Geometry check sheet. Reference: the model listing, model coordinates, mm. Face numbers are marked on the shaded views. Coordinates: 2 decimals unless noted, no trailing zeros. Order: outer loops, then holes, each group sorted by start corner. A loop starts at its lowest first (then second) coordinate and runs counter-clockwise, first axis right, second up. Notation, with made-up numbers: M 27.25,-27.75 L 72.25,-27.75 A11 cw 72.25,-10.75 Z; hole C 80.5,-19 d5. An arc over 180 degrees is marked long. One line per item, written item: value. Start each with the question number.
1) Thickness scan on L1, parallel to Z at x = -60.5, y = 8; L2, parallel to Z at x = -73, y = 5.5; L3, parallel to Y at x = -23.5, z = -3.5. Record the ranges inside material, lowest first. Write a range as from..to.
2) Sectioned sample at B-B, the plane z = -13.75. Enter the section's corners in (x, y), then the cut area to 3 significant figures.
3) Go/stop test with flat-tipped pins: P1, Ø12, axis at x = 75.5, y = -13.5, coming from the -Z side; P2, Ø2.5, axis at x = -84.5, y = 21, coming from the -Z side; P3, Ø3.5, axis at x = -101, y = -3.5, coming from the +Z side. Record where each tip stops, or that it passes through.
4) Draft check along X on the marked faces 1, 2 and 3. Enter one of: pulls with the +X half, pulls with the -X half, needs draft (parallel to the pull), parting line crosses it, or undercut.
5) Sectioned sample at A-A, the plane z = 0. Enter the section's corners in (x, y), then the cut area to 3 significant figures.
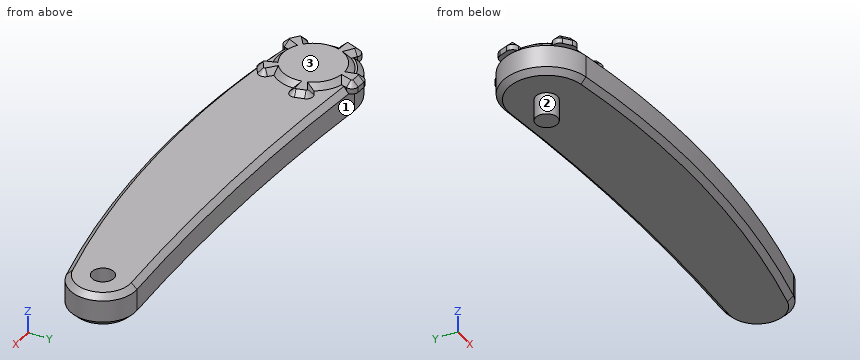
```python
from build123d import *

# Parameters (mm, degrees)
BOSS_EXTRUDE2_DEPTH = 7.5
CHAMFER1_SIZE       = 2.5
SKETCH4_R           = 16.5
BOSS_EXTRUDE3_DEPTH = 2.5
BOSS_EXTRUDE4_DEPTH = 5
CHAMFER2_SIZE       = 2.5
SKETCH6_R           = 5
CUT_EXTRUDE1_DEPTH  = 10
SKETCH7_R           = 5
BOSS_EXTRUDE5_DEPTH = 10


with BuildPart() as part:
    # Sketch1 → Boss-Extrude2 (new, symmetric)
    with BuildSketch(Plane.XY):
        with BuildLine():
            ThreePointArc((84.460518945, 14.977598104), (0.616073919, 13.910903957), (-83.022979725, 19.872238008))
            ThreePointArc((-83.022979725, 19.872238008), (-105.080474764, 2.818038301), (-88.656802688, -19.712869593))
            ThreePointArc((-88.656802688, -19.712869593), (0.254242747, -25.987416271), (88.657894096, -14.614713664))
            ThreePointArc((88.657894096, -14.614713664), (100.131353297, 2.106516275), (84.460518945, 14.977598104))
        make_face()
    extrude(amount=BOSS_EXTRUDE2_DEPTH, both=True)

    # Chamfer1
    chamfer1_edges = [part.edges().sort_by_distance(p)[0] for p in [
        (100.131353297, 2.106516275, 7.5),
        (0.616073919, 13.910903957, 7.5),
        (-105.080474764, 2.818038301, 7.5),
        (0.254242747, -25.987416271, 7.5),
        (-105.080474764, 2.818038301, -7.5),
        (0.616073919, 13.910903957, -7.5),
        (100.131353297, 2.106516275, -7.5),
        (0.254242747, -25.987416271, -7.5),
    ]]
    chamfer(chamfer1_edges, length=CHAMFER1_SIZE)

    # Sketch4 → Boss-Extrude3 (add, symmetric)
    with BuildSketch(Plane.XY.offset(7.5)):
        with Locations((-85.280003554, 0)):
            Circle(SKETCH4_R)
    extrude(amount=BOSS_EXTRUDE3_DEPTH, both=True)

    # Sketch5 → Boss-Extrude4 (add)
    with BuildSketch(Plane.XY.offset(10)):
        with BuildLine():
            Line((-68.665882393, 9.592167325), (-85.280003554, 0))
            Line((-85.280003554, 0), (-66.095668905, 0))
            ThreePointArc((-66.095668905, 0), (-63.715608884, 1.173715713), (-63.197891426, 3.776457135))
            Line((-63.197891426, 3.776457135), (-64.268104914, 7.770548248))
            ThreePointArc((-64.268104914, 7.770548248), (-66.017832096, 9.765729711), (-68.665882393, 9.592167325))
        make_face()
        with BuildLine():
            Line((-71.023264529, -12.836825476), (-85.280003554, 0))
            Line((-85.280003554, 0), (-79.351718121, -18.245386479))
            ThreePointArc((-79.351718121, -18.245386479), (-77.49996915, -20.146259969), (-74.864631467, -19.834347199))
            Line((-74.864631467, -19.834347199), (-71.396739243, -17.582271657))
            ThreePointArc((-71.396739243, -17.582271657), (-70.039904347, -15.30163724), (-71.023264529, -12.836825476))
        make_face()
        with BuildLine():
            Line((-93.082975429, -17.525761777), (-85.280003554, 0))
            Line((-85.280003554, 0), (-100.800456311, -11.276268982))
            ThreePointArc((-100.800456311, -11.276268982), (-102.036072529, -13.62478912), (-100.925061727, -16.034757849))
            Line((-100.925061727, -16.034757849), (-97.711572975, -18.636989732))
            ThreePointArc((-97.711572975, -18.636989732), (-95.12327571, -19.222661609), (-93.082975429, -17.525761777))
        make_face()
        with BuildLine():
            Line((-104.35924441, 2.00530902), (-85.280003554, 0))
            Line((-85.280003554, 0), (-100.800456311, 11.276268982))
            ThreePointArc((-100.800456311, 11.276268982), (-103.415858102, 11.725677203), (-105.364553347, 9.924321847))
            Line((-105.364553347, 9.924321847), (-106.8464003, 6.063978554))
            ThreePointArc((-106.8464003, 6.063978554), (-106.603579514, 3.421379012), (-104.35924441, 2.00530902))
        make_face()
        with BuildLine():
            Line((-89.268651008, 18.765110909), (-85.280003554, 0))
            Line((-85.280003554, 0), (-79.351718121, 18.245386479))
            ThreePointArc((-79.351718121, 18.245386479), (-79.732509104, 20.871656173), (-82.047879802, 22.168326066))
            Line((-82.047879802, 22.168326066), (-86.177200337, 22.384734585))
            ThreePointArc((-86.177200337, 22.384734585), (-88.615426102, 21.337190126), (-89.268651008, 18.765110909))
        make_face()
    extrude(amount=-BOSS_EXTRUDE4_DEPTH)

    # Chamfer2
    chamfer2_edges = [part.edges().sort_by_distance(p)[0] for p in [
        (-69.828233392, 8.921083662, 10),
        (-66.017832096, 9.765729711, 10),
        (-63.73299817, 5.773502692, 10),
        (-63.715608884, 1.173715713, 10),
        (-67.437836229, 0, 10),
        (-69.875926517, -5.913071167, 10),
        (-72.020689231, -11.938740241, 10),
        (-70.039904347, -15.30163724, 10),
        (-73.130685355, -18.708309428, 10),
        (-77.49996915, -20.146259969, 10),
        (-79.766470634, -16.968909499, 10),
        (-86.143546832, -16.477387323, 10),
        (-92.537066797, -16.299630914, 10),
        (-95.12327571, -19.222661609, 10),
        (-99.318317351, -17.33587379, 10),
        (-102.036072529, -13.62478912, 10),
        (-99.714620136, -10.487362822, 10),
        (-101.217779688, -4.270514244, 10),
        (-103.024429619, 1.865014332, 10),
        (-106.603579514, 3.421379012, 10),
        (-106.105476824, 7.994150201, 10),
        (-103.415858102, 11.725677203, 10),
        (-99.714620136, 10.487362822, 10),
        (-94.266547632, 13.838064371, 10),
        (-88.98959873, 17.45227316, 10),
        (-88.615426102, 21.337190126, 10),
        (-84.112540069, 22.276530326, 10),
        (-79.732509104, 20.871656173, 10),
        (-79.766470634, 16.968909499, 10),
        (-74.896217101, 12.822908364, 10),
    ]]
    chamfer(chamfer2_edges, length=CHAMFER2_SIZE - 0.0001)  # a hair under: the kernel refuses the full size

    # Sketch6 → Cut-Extrude1 (cut)
    with BuildSketch(Plane.XY.offset(7.5)):
        with Locations((85.280003554, 0)):
            Circle(SKETCH6_R)
    extrude(amount=-CUT_EXTRUDE1_DEPTH, mode=Mode.SUBTRACT)

    # Sketch7 → Boss-Extrude5 (add)
    with BuildSketch(Plane(origin=(0, 0, -7.5), x_dir=(-1, 0, 0), z_dir=(0, 0, -1))):
        with Locations((85.280003554, 0)):
            Circle(SKETCH7_R)
    extrude(amount=BOSS_EXTRUDE5_DEPTH)


solid = part.part
```
Final values:
1. L1: z = -7.5..7.5
1. L2: z = -7.5..10
1. L3: y = -26.04..14.91
2. outline: C -85.28,0 d10
2. area: 78.5 mm^2
3. P1: stops at z = -7.5
3. P2: stops at z = -5.24
3. P3: stops at z = 9.65
4. face 1: undercut
4. face 2: parting line crosses it
4. face 3: needs draft
5. outline: M -88.66,-19.71 A450 ccw 88.66,-14.61 A15 ccw 84.46,14.98 A1000 cw -83.02,19.87 A20 ccw Z; hole C 85.28,0 d10
5. area: 7,460 mm^2
